from build123d import *

# Parameters (mm, degrees)
SKETCH_1_W          = 100
SKETCH_1_H          = 100
EXTRUDE_1_DEPTH     = 7
FILLET_1_R          = 10
SKETCH_2_R          = 1.52
SKETCH_2_R_2        = 2.02
CUT_EXTRUDE_2_DEPTH = 13


with BuildPart() as part:
    # 草图1 → 凸台-拉伸1 (new body)
    with BuildSketch(Plane(origin=(0, 0, 0), x_dir=(1, 0, 0), z_dir=(0, 1, 0))):
        with Locations((50, 50)):
            Rectangle(SKETCH_1_W, SKETCH_1_H)
    extrude(amount=EXTRUDE_1_DEPTH)

    # 圆角1
    fillet_1_edges = [part.edges().sort_by_distance(p)[0] for p in [
        (0, 3.5, 0),
        (0, 3.5, -100),
        (100, 3.5, -100),
        (100, 3.5, 0),
    ]]
    fillet(fillet_1_edges, radius=FILLET_1_R)

    # 草图2 → 切除-拉伸2 (cut)
    with BuildSketch(Plane(origin=(0, 7, 0), x_dir=(1, 0, 0), z_dir=(0, 1, 0))):
        with BuildLine():
            ThreePointArc((22.02, 79.5), (21.574802307, 80.574802307), (20.5, 81.02))
            Line((20.5, 81.02), (20.5, 79.5))
            Line((20.5, 79.5), (18.98, 79.5))
            ThreePointArc((18.98, 79.5), (20.5, 77.98), (22.02, 79.5))
        make_face()
        with BuildLine():
            Line((20.5, 79.5), (20.5, 81.02))
            ThreePointArc((20.5, 81.02), (19.425197693, 80.574802307), (18.98, 79.5))
            Line((18.98, 79.5), (20.5, 79.5))
        make_face()
        with BuildLine():
            ThreePointArc((6.02, 79.5), (4, 81.52), (1.98, 79.5))
            Line((1.98, 79.5), (4, 79.5))
            Line((4, 79.5), (6.02, 79.5))
        make_face()
        with BuildLine():
            Line((4, 79.5), (1.98, 79.5))
            ThreePointArc((1.98, 79.5), (4, 77.48), (6.02, 79.5))
            Line((6.02, 79.5), (4, 79.5))
        make_face()
        with BuildLine():
            ThreePointArc((22.52, 96), (21.928355698, 97.428355698), (20.5, 98.02))
            Line((20.5, 98.02), (20.5, 96))
            Line((20.5, 96), (20.5, 93.98))
            ThreePointArc((20.5, 93.98), (21.928355698, 94.571644302), (22.52, 96))
        make_face()
        with BuildLine():
            Line((20.5, 96), (20.5, 98.02))
            ThreePointArc((20.5, 98.02), (18.48, 96), (20.5, 93.98))
            Line((20.5, 93.98), (20.5, 96))
        make_face()
        with Locations((79.5, 79.5)):
            Circle(SKETCH_2_R)
        with Locations((79.5, 96)):
            Circle(SKETCH_2_R_2)
        with Locations((96, 79.5)):
            Circle(SKETCH_2_R_2)
        with Locations((79.5, 20.5)):
            Circle(SKETCH_2_R)
        with Locations((96, 20.5)):
            Circle(SKETCH_2_R_2)
        with Locations((79.5, 4)):
            Circle(SKETCH_2_R_2)
        with Locations((20.5, 20.5)):
            Circle(SKETCH_2_R)
        with Locations((4, 20.5)):
            Circle(SKETCH_2_R_2)
        with Locations((20.5, 4)):
            Circle(SKETCH_2_R_2)
    extrude(amount=-CUT_EXTRUDE_2_DEPTH, mode=Mode.SUBTRACT)


solid = part.part
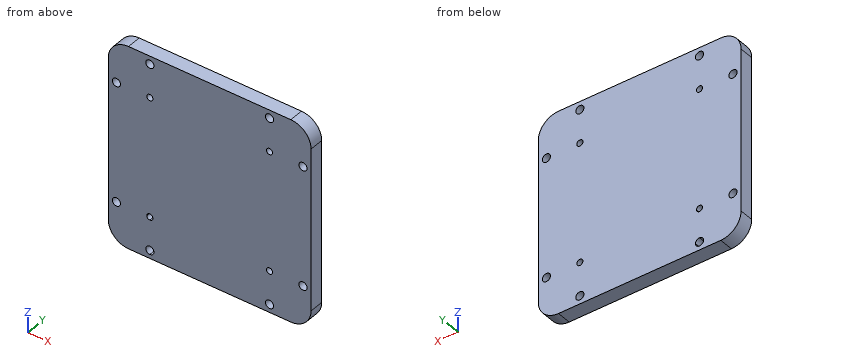
Design review of the part built by this model. Coordinates are the model's own, in mm. Coordinates: 2 decimals unless noted, no trailing zeros. Order: outer loops, then holes, each group sorted by start corner. A loop starts at its lowest first (then second) coordinate and runs counter-clockwise, first axis right, second up. Notation, with made-up numbers: (40, 75.25) -> (45, 75.25) arc R7 ccw to (45, 82.25) -> close; hole circle Ø6 at (44, 44.25). An arc over 180 degrees is marked (long way). Use one line per item in the form item = value. Start each with the question number.
(1) Insertion check: pin 1 (3.5 mm diameter, centred on x = 4, z = -20.5, fed in from -Y). The pin has a flat end and moves straight along its axis. Give the tip position at first contact, or say it passes through.
(2) Add section A-A on z = -20.5. State the section outline as (x, y) points.
(3) Add section B-B on x = 96. State the section outline as (y, z) points.
(4) Add section C-C on y = 2.25. Give the number of separate pieces and of enclosed holes in the cut face, plus the area to 3 significant figures.
(5) For probe 1 along Z at (x, y) = (96, 3.5); probe 2 along X at (y, z) = (2, -96); probe 3 along X at (y, z) = (4, -79.5), list the stretches that pass through material, from the lowest coordinate up.
(6) Add section D-D on x = 79.5. State the section outline as (y, z) points, plus the area to 3 significant figures.
Answer block:
q1.pin_1 = through
q2.outline = (0, 0) -> (1.98, 0) -> (1.98, 7) -> (0, 7) -> close; (6.02, 0) -> (18.98, 0) -> (18.98, 7) -> (6.02, 7) -> close; (22.02, 0) -> (77.98, 0) -> (77.98, 7) -> (22.02, 7) -> close; (81.02, 0) -> (93.98, 0) -> (93.98, 7) -> (81.02, 7) -> close; (98.02, 0) -> (100, 0) -> (100, 7) -> (98.02, 7) -> close
q3.outline = (0, -98) -> (7, -98) -> (7, -81.52) -> (0, -81.52) -> close; (0, -77.48) -> (7, -77.48) -> (7, -22.52) -> (0, -22.52) -> close; (0, -18.48) -> (7, -18.48) -> (7, -2) -> (0, -2) -> close
q4.separate_pieces = 1
q4.enclosed_holes = 12
q4.area = 9,780 mm²
q5.probe_1 = -98 to -81.52, -77.48 to -22.52, -18.48 to -2
q5.probe_2 = 2 to 18.48, 22.52 to 77.48, 81.52 to 98
q5.probe_3 = 0 to 1.98, 6.02 to 18.98, 22.02 to 77.98, 81.02 to 93.98, 98.02 to 100
q6.outline = (0, -100) -> (7, -100) -> (7, -98.02) -> (0, -98.02) -> close; (0, -93.98) -> (7, -93.98) -> (7, -81.02) -> (0, -81.02) -> close; (0, -77.98) -> (7, -77.98) -> (7, -22.02) -> (0, -22.02) -> close; (0, -18.98) -> (7, -18.98) -> (7, -6.02) -> (0, -6.02) -> close; (0, -1.98) -> (7, -1.98) -> (7, 0) -> (0, 0) -> close
q6.area = 601 mm²
